Verification items for the finished model (mm, model axes). A direction names the side the tool comes from. Coordinates: 2 decimals unless noted, no trailing zeros. Order: outer loops, then holes, each group sorted by start corner. A loop starts at its lowest first (then second) coordinate and runs counter-clockwise, first axis right, second up. Notation, with made-up numbers: (28.5, 80) -> (84.5, 80) arc R31 ccw to (84.5, 119) -> close; hole circle Ø9 at (53, 13). An arc over 180 degrees is marked (long way). Write item = value, one per line. Start each with the question number.
1. Go/stop test with flat-tipped pins: P1, Ø1.1, axis at x = -1.5, z = 0.5, coming from the +Y side; P2, Ø1.6, axis at x = -2, z = 0, coming from the -Y side; P3, Ø1.5, axis at x = 6.5, y = 2, coming from the -Z side. Record where each tip stops, or that it passes through.
2. Cross-section at A-A on x = 11.25. Record the cut outline in (y, z).
3. Set-up check for faces 1 (the flat face through (-2, 1.25, 0)), 2 (the flat face through (16, 0, 0)): record each of +Z, -Z, +X, -X, +Y, -Y from which the full face is reachable in a straight line by a thin tool's end or side.
4. Release check for a two-part mould opening along Y. For faces 3 (the flat face through (-1.504, 0.616, -1.088)), 4 (the cylindrical face through (8, 0, 2)), 5 (the flat face through (0, 2, -2)) record: +Y half, -Y half, draft (parallel to the pull), parting line (faces both ways), or undercut.
5. Thickness scan on line 1 along Z through (x, y) = (13.25, 0); line 2 along X through (y, z) = (3.5, -1); line 3 along Z through (x, y) = (9, -1). Record the ranges inside material, lowest first. Write a range as from..to.
Autodesk Inventor part; units mm, degrees
ref_plane "Work Plane1" through (29, 0, 0) normal (0, -1, 0) x (1, 0, 0)
ref_plane "YZ Plane" through (0, 0, 0) normal (1, 0, 0) x (0, 1, 0)
ref_plane "XZ Plane" through (0, 0, 0) normal (0, 1, 0) x (-1, 0, 0)
sketch "Эскиз1" plane through (0, 0, 0) normal (0, 0, 1) x (1, 0, 0)
  line L0 (-0.0667, 0) -> (16, 0)
  line L1 (16, 0) -> (16, 2)
  line L2 (16, 2) -> (1.4, 2)
  line L3 (1.4, 2) -> (0.9705, 2)
  line L4 (0.9705, 2) -> (0, 2)
  line L5 (0, 2) -> (0, 3.8)
  line L6 (0, 3.8) -> (-2.2, 3.8)
  line L7 (-2.2, 3.8) -> (-2.2, 1.4434)
  line L8 (-2.2, 1.4434) -> (-0.9, 1.4434)
  line L9 (-0.9, 1.4434) -> (-0.0667, 0)
  line L10 (-5.84, 0) -> (19.64, 0)
  line L11 (0, -0.76) -> (0, 4.56)
  line L12 (1.4, 2) -> (0, 2) construction
  dimension "d1" = 14.6
  dimension "d2" = 0.4295
  dimension "d3" = 2.2
  dimension "d4" = 1.3
  dimension "d5" = 60
  dimension "d6" = 4
  dimension "d7" = 4
  dimension "d8" = 2.8868
  dimension "d9" = 7.6
  dimension "d26" = 16
revolve "Базовый элемент" add sketch "Эскиз1" angle 360 about axis through (-0.0667, 0, 0) along (1, 0, 0)
sketch "Эскиз2" plane through (-2.2, 0, 0) normal (-1, 0, 0) x (0, 0, 1)
  circle A0 centre (0, 0) radius 1.4434
  line L0 (0, -5.32) -> (0, 5.32)
  line L1 (-5.32, 0) -> (5.32, 0)
  line L2 (1.4434, 0) -> (0.7217, -1.25)
  line L3 (0.7217, -1.25) -> (-0.7217, -1.25)
  line L4 (-0.7217, -1.25) -> (-1.4434, 0)
  line L5 (-1.4434, 0) -> (-0.7217, 1.25)
  line L6 (-0.7217, 1.25) -> (0.7217, 1.25)
  line L7 (0.7217, 1.25) -> (1.4434, 0)
  point P0 (0, 0)
extrude "Паз" add sketch "Эскиз2" against normal up to next contours L7 A0 | A0 L2 | L6 L0 A0 | A0 L0 L3 | L0 L6 A0 | A0 L3 L0 | L4 A0 | A0 L5
fillet "Сопряжение1" radius 1.87 1 edges at (-2.2, -3.8, 0)
thread "Резьба"
chamfer "Фаска1" distance 0.4294 distance2 0.4294 1 edges at (16, -2, 0) measured on face at (16, 0.527, -0.2661)
ref_plane "Work Plane1" through (29, 0, 0) normal (0, -1, 0) x (1, 0, 0)
fillet "Fillet2" radius 0.1 1 edges at (0, -2, 0)
equation "\"d1\" = GEL"
equation "\"d3\" = KOH"
equation "\"d4\" = INTI"
equation "\"d6\" = GD"
equation "\"d7\" = BDM"
equation "\"d8\" = 1.1547 * SW"
equation "\"d9\" = KOD"
equation "\"d26\" = NLG"
equation "\"d30\" = R"
equation "\"d17\" = RR"
equation "\"d13\" = GEL"
equation "\"d15\" = -0.5 * SPD + 0.5 * GD"
equation "\"d16\" = GUL"
equation "\"GD\" = NND"
equation "\"NLG\" = 16"
equation "\"GEL\" = 14.6"
equation "\"KOD\" = 7.6"
equation "\"KOH\" = 2.2"
equation "\"INTI\" = 1.3"
equation "\"GAL\" = 0.61345 * PTC"
equation "\"GUL\" = 0.61345 * PTC"
equation "\"BDM\" = NND"
equation "\"SW\" = 2.5"
equation "\"RR\" = 1.87"
equation "\"SPD\" = 3.14117"
equation "\"R\" = 0.1"
equation "\"TOA\" = 30deg"
equation "\"GD1\" = THREADDIA - 1.2269 * PTC"
equation "\"THREADDIA\" = 4"
equation "\"PTC\" = 0.7"
equation "\"NND\" = 4"
equation "\"E0\" = 2.87"
properties part number "JIS B 1174 - M4 x 16" material "Сталь, мягкая"
Worked out:
q1.P1 = 3.67
q1.P2 = -3.59
q1.P3 = -1.56
q2.outline = circle Ø4 at (0, 0)
q3.face_1 = -X
q3.face_2 = +Z, -Z, +X, +Y, -Y
q4.face_3 = undercut
q4.face_4 = parting line
q4.face_5 = draft
q5.line_1 = -2..2
q5.line_2 = -1.09..0
q5.line_3 = -1.73..1.73
